```python
from build123d import *

# Parameters (mm, degrees)
F1_DEPTH = 38.1
F2_R     = 2.54


with BuildPart() as f1:
    # F0 (on Front) → F1 (new body)
    with BuildSketch(Plane.XZ):
        with BuildLine():
            Line((0, -82.55), (-62.818537, -28.993171))
            ThreePointArc((-62.818537, -28.993171), (-72.693253, -15.966117), (-76.2, 0))
            ThreePointArc((-76.2, 0), (-90.414977, 61.72931), (-38.1, 97.446484))
            ThreePointArc((-38.1, 97.446484), (-129.539011, 33.685671), (-101.317971, -74.157302))
            Line((-101.317971, -74.157302), (0, -165.1))
            Line((0, -165.1), (0, -82.55))
        make_face()
        with BuildLine():
            ThreePointArc((76.2, 0), (72.693253, -15.966117), (62.818537, -28.993171))
            Line((62.818537, -28.993171), (0, -82.55))
            Line((0, -82.55), (0, -165.1))
            Line((0, -165.1), (101.317932, -74.157335))
            ThreePointArc((101.317932, -74.157335), (129.53902, 33.685647), (38.1, 97.446484))
            ThreePointArc((38.1, 97.446484), (77.819237, 80.994237), (94.271484, 41.275))
            ThreePointArc((94.271484, 41.275), (89.555656, 18.746107), (76.2, 0))
        make_face()
        with BuildLine():
            ThreePointArc((18.071484, 41.275), (17.874678, 36.577013), (17.285638, 31.911946))
            ThreePointArc((17.285638, 31.911946), (28.71095, 36.925002), (41.143131, 37.978275))
            ThreePointArc((41.143131, 37.978275), (66.096011, 25.842472), (76.2, 0))
            ThreePointArc((76.2, 0), (89.555656, 18.746107), (94.271484, 41.275))
            ThreePointArc((94.271484, 41.275), (77.819237, 80.994237), (38.1, 97.446484))
            ThreePointArc((38.1, 97.446484), (17.64569, 93.589977), (0, 82.55))
            ThreePointArc((0, 82.55), (13.355656, 63.803893), (18.071484, 41.275))
        make_face()
        with BuildLine():
            ThreePointArc((-17.285638, 31.911946), (-4.598976, 18.146388), (0, 0))
            Line((0, 0), (0, 82.55))
            ThreePointArc((0, 82.55), (-15.059611, 59.421388), (-17.285638, 31.911946))
        make_face()
        with BuildLine():
            Line((0, 82.55), (0, 0))
            ThreePointArc((0, 0), (4.598976, 18.146388), (17.285638, 31.911946))
            ThreePointArc((17.285638, 31.911946), (17.874678, 36.577013), (18.071484, 41.275))
            ThreePointArc((18.071484, 41.275), (13.355656, 63.803893), (0, 82.55))
        make_face()
        with BuildLine():
            ThreePointArc((-41.143131, 37.978275), (-28.71095, 36.925002), (-17.285638, 31.911946))
            ThreePointArc((-17.285638, 31.911946), (-15.059611, 59.421388), (0, 82.55))
            ThreePointArc((0, 82.55), (-17.64569, 93.589977), (-38.1, 97.446484))
            ThreePointArc((-38.1, 97.446484), (-90.414977, 61.72931), (-76.2, 0))
            ThreePointArc((-76.2, 0), (-66.096011, 25.842472), (-41.143131, 37.978275))
        make_face()
    extrude(amount=F1_DEPTH)

    # F2
    f2_edges = [f1.edges().sort_by_distance(p)[0] for p in [
        (0, -19.05, 0),
    ]]
    fillet(f2_edges, radius=F2_R)


solid = f1.part
```
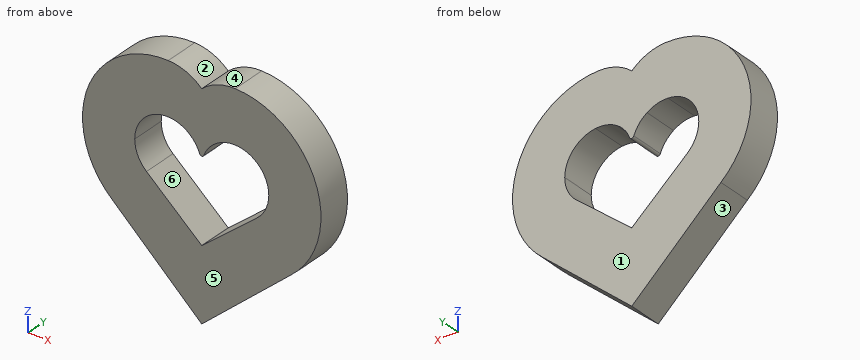
Source: CAD feature listing. Evaluate the final solid. Frame: model axes, mm. Face numbers are marked on the shaded views. A direction names the side the tool comes from. Give positions to 0.01 mm unless a question says otherwise; leave off trailing zeros. Loops run counter-clockwise (first coordinate to the right, second up) from the corner with the lowest first, then second, coordinate; pieces in that order, holes last. Notation, with made-up numbers: (-10, 35) -> (39, 35) arc R26 cw to (39, 64) -> close; hole circle Ø10 at (69, 71.5). An arc over 180 degrees is marked (long way). Use a Markdown table: item, result. Add a question column.
(1) Ray query, line 1 (X direction, y = -2.5, z = 26); line 2 (Z direction, x = -46.5, y = -11.5); line 3 (Z direction, x = 48.5, y = -10). Return the intervals inside material, ascending.
(2) Section query A-A (z = -69). Output: boundary loops of the cut face in (x, y), then the cut area to 3 significant figures.
(3) Access query for the marked faces 1 and 2. Directions: +Z, -Z, +X, -X, +Y, -Y. A direction counts if a zero-diameter tool reaches every point of the face in a straight line with its end or side. Return the directions, or none.
(4) First-contact query: pin 1 Ø4 at (y, z) = (-30.5, -57) entering from +X; pin 2 Ø6 at (y, z) = (-19.5, -117.5) entering from +X; pin 3 Ø12 at (y, z) = (-22.5, -94) entering from +X. Flat tips, straight axial feed; report the tip coordinate or a pass-through.
(5) Pull-direction query (Z, two-part tool) for the marked faces 3, 4, 5 and 6; classes: +Z half, -Z half, draft (parallel to the pull), parting line (faces both ways), or undercut.
(6) Section query D-D (z = -135). Output: boundary loops of the cut face in (x, y), then the cut area to 3 significant figures.
(7) Section query B-B (x = 68.5). Output: boundary loops of the cut face in (y, z), then the cut area to 3 significant figures.
(8) Section query C-C (x = -94.5). Output: boundary loops of the cut face in (y, z).
Checked values:
| question | item | result |
|---|---|---|
| 1 | line 1 | -132.01 to -65.95, -10.25 to 10.25, 65.95 to 132.01 |
| 1 | line 2 | -123.36 to -42.91, 37.16 to 97.08 |
| 1 | line 3 | -121.57 to -41.2, 36.65 to 96.89 |
| 2 | outline | (-106.91, -38.1) -> (-15.89, -38.1) -> (-15.89, 0) -> (-106.91, 0) -> close; (15.89, -38.1) -> (106.91, -38.1) -> (106.91, 0) -> (15.89, 0) -> close |
| 2 | area | 6,940 mm^2 |
| 3 | face 1 | +Z, -Z, +X, -X, +Y |
| 3 | face 2 | +Z, +Y, -Y |
| 4 | pin 1 | x = 118.54 |
| 4 | pin 2 | x = 56.37 |
| 4 | pin 3 | x = 85.9 |
| 5 | face 3 | -Z half |
| 5 | face 4 | +Z half |
| 5 | face 5 | draft |
| 5 | face 6 | undercut |
| 6 | outline | (-33.53, -38.1) -> (33.53, -38.1) -> (33.53, 0) -> (-33.53, 0) -> close |
| 6 | area | 2,560 mm^2 |
| 7 | outline | (-38.1, -103.61) -> (0, -103.61) -> (0, -22.97) -> (-38.1, -22.97) -> close; (-38.1, 22.97) -> (0, 22.97) -> (0, 92.58) -> (-38.1, 92.58) -> close |
| 7 | area | 5,730 mm^2 |
| 8 | outline | (-38.1, -80.28) -> (0, -80.28) -> (0, 79.47) -> (-38.1, 79.47) -> close |
